Verification items for this drawing (mm, ordinates from the low corner). A direction names the side the tool comes from. Coordinates: 2 decimals unless noted, no trailing zeros. Write each loop counter-clockwise with the first axis right and the second up, starting at its lowest first coordinate (ties: lowest second). Pieces come first, ordered by that corner, then holes. Notation, with made-up numbers: (50.5, 36) -> (102.5, 36) arc R34 cw to (102.5, 66) -> close; hole circle Ø6 at (14, 34.25). An arc over 180 degrees is marked (long way). Put each result on its own line as item: value. Start each with the question number.
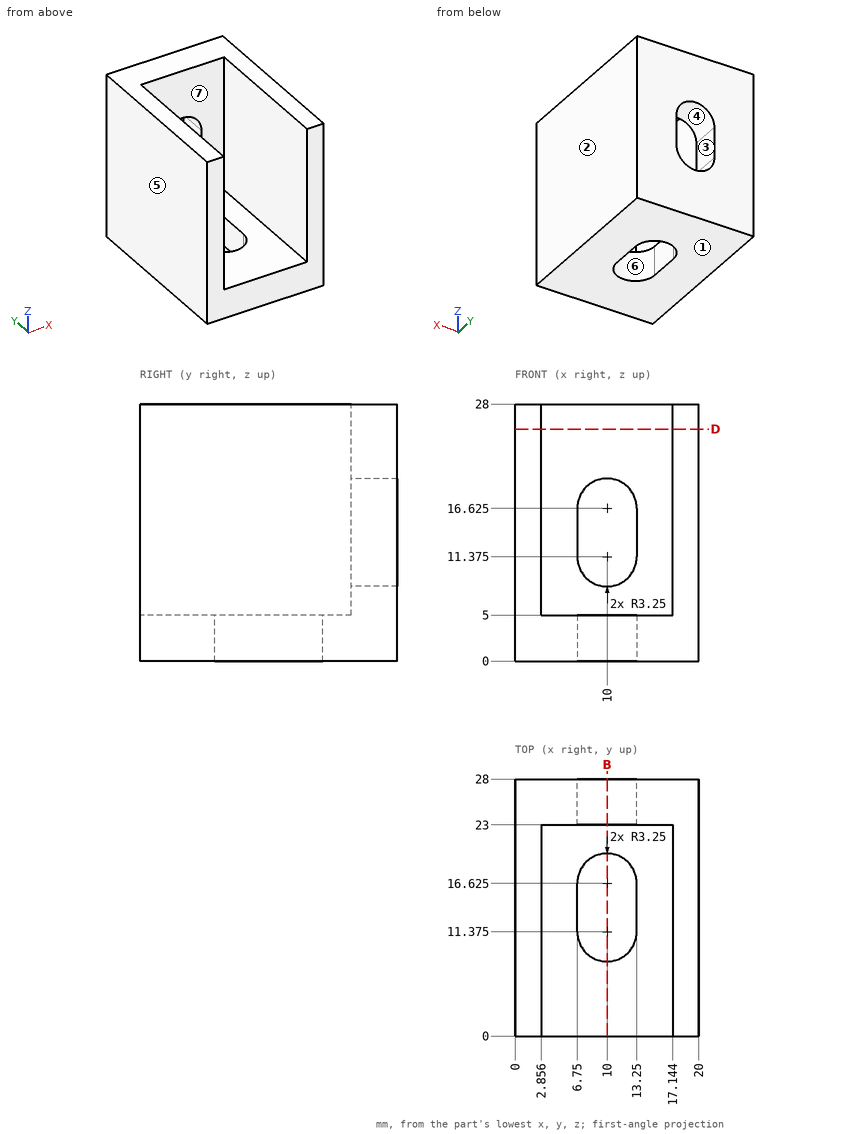
Item 1: Go/stop test with flat-tipped pins: P1, Ø4.5, axis at x = 7, y = 6, coming from the +Z side; P2, Ø1.5, axis at x = 11, y = 21, coming from the -Z side. Record where each tip stops, or that it passes through.
Item 2: Scan lines: line 1 along X through (y, z) = (14, 3); line 2 along X through (y, z) = (14.75, 21) (1 decimal); line 3 along Y through (x, z) = (4.5, 7). Record each from-to range of solid material in increasing order. Write a range as [from, to].
Item 3: Mould release check, pull along Z, two halves, no side actions. Record for the marked faces 1, 2, 3 and 4: released by +Z, released by -Z, zero draft, split by the parting line, or undercut.
Item 4: Section check D-D, the plane z = 25.25. Enter the section's corners in (x, y) (1 decimal).
Item 5: Access from +Z, -Z, +X, -X, +Y, -Y to the whole of each face (thin tool, end or side, straight path). Record for the marked faces 5, 6 and 7.
Item 6: Section check B-B, the plane x = 10. Enter the section's corners in (y, z) (1 decimal).
From the geometry:
1. P1: z = 5
1. P2: z = 0
2. line 1: [0, 6.75], [13.25, 20]
2. line 2: [0, 2.9], [17.1, 20]
2. line 3: [23, 28]
3. face 1: released by -Z
3. face 2: zero draft
3. face 3: undercut
3. face 4: undercut
4. outline: (0, 0) -> (2.9, 0) -> (2.9, 23) -> (17.1, 23) -> (17.1, 0) -> (20, 0) -> (20, 28) -> (0, 28) -> close
5. face 5: +Z, -Z, -X, +Y, -Y
5. face 6: +Z, -Z
5. face 7: +Z, -Y
6. outline: (0, 0) -> (8.1, 0) -> (8.1, 5) -> (0, 5) -> close; (19.9, 0) -> (28, 0) -> (28, 8.1) -> (23, 8.1) -> (23, 5) -> (19.9, 5) -> close; (23, 19.9) -> (28, 19.9) -> (28, 28) -> (23, 28) -> close
